Could you check a few things on this model? Use its own coordinates, in mm. A direction names the side the tool comes from. Give positions to 0.01 mm unless a question says otherwise; leave off trailing zeros. Loops run counter-clockwise (first coordinate to the right, second up) from the corner with the lowest first, then second, coordinate; pieces in that order, holes last.
1. Imagine slicing it at D-D (z = -13). List the corners of the cut face in (x, y) for me, plus the area to 3 significant figures.
2. I need wall thicknesses on line 1 along X through (y, z) = (1.75, -7.25) (3 decimals); line 2 along X through (y, z) = (1.15, 7.65) (3 decimals); line 3 along Z through (x, y) = (-15.6, 1.4) (3 decimals). Which ranges of each line are inside material? Lowest first, please.
3. Imagine slicing it at A-A (x = -9). List the corners of the cut face in (y, z) for me, plus the area to 3 significant figures.
4. For P1, Ø1.2, axis at x = -15.6, z = -7.25, coming from the -Y side; P2, Ø1.5, axis at x = 18.5, y = 9, coming from the -Z side; P3, Ø3, axis at x = -14, y = 10, coming from the -Z side, each with a flat end and sliding along its axis, tell me the tip position at first contact or that it passes through.
5. Thinking about a two-plate mould opening in X: for faces 3 (the cylindrical face through (-19.65, 1.23, 15.24)), 4 (the cylindrical face through (19.65, 1.23, -15.24)), 5 (the cylindrical face through (15.05, 1.52, 8.04)), which applies, +X half, -X half, draft (parallel to the pull), parting line (faces both ways), or undercut?
6. Imagine slicing it at C-C (z = 0). List the corners of the cut face in (x, y) for me.
7. Imagine slicing it at B-B (y = 8.25). List the corners of the cut face in (x, z) for me, plus the area to 3 significant figures.
8. For faces 1 (the cylindrical face through (0.18, 9.65, -15.24)), 2 (the cylindrical face through (-14.65, 1.52, -6.86)), which set-ups out of +Z, -Z, +X, -X, +Y, -Y let a thin tool reach every point of the face, with its end or its side?
```python
from build123d import *

# Parameters (mm, degrees)
SKETCH1_W                          = 45
SKETCH1_H                          = 36.5
BOSS_EXTRUDE1_DEPTH                = 12.5
SKETCH2_R                          = 1.375
BOSS_EXTRUDE2_DEPTH                = 1
TAP_DRILL_FOR_M2_5X0_45_TAP1_D     = 2.05
TAP_DRILL_FOR_M2_5X0_45_TAP1_DEPTH = 3
TAP_DRILL_FOR_M2_5X0_45_TAP1_TIP   = 0.615882135
FILLET1_R                          = 10


with BuildPart() as part:
    # Sketch1 → Boss-Extrude1 (new body)
    with BuildSketch(Plane(origin=(0, 0, 0), x_dir=(1, 0, 0), z_dir=(0, 1, 0))):
        Rectangle(SKETCH1_W, SKETCH1_H)
    extrude(amount=BOSS_EXTRUDE1_DEPTH)

    # Sketch2 → Boss-Extrude2 (add)
    with BuildSketch(Plane(origin=(22.5, 0, 0), x_dir=(0, 0, -1), z_dir=(1, 0, 0))):
        with Locations(Location((0, 5.884601179, 0), (0, 0, 180))):
            Circle(SKETCH2_R)
    extrude(amount=BOSS_EXTRUDE2_DEPTH)

    # Tap Drill for M2.5x0.45 Tap1
    with Locations(Plane(origin=(0, 0, 0), x_dir=(-1, 0, 0), z_dir=(0, -1, 0))):
        with Locations((15.6, 7.25), (-14.1, -7.65)):
            Hole(TAP_DRILL_FOR_M2_5X0_45_TAP1_D / 2, depth=TAP_DRILL_FOR_M2_5X0_45_TAP1_DEPTH)
            with Locations((0, 0, -(TAP_DRILL_FOR_M2_5X0_45_TAP1_DEPTH + TAP_DRILL_FOR_M2_5X0_45_TAP1_TIP / 2))):  # 118° drill point
                Cone(0, TAP_DRILL_FOR_M2_5X0_45_TAP1_D / 2, TAP_DRILL_FOR_M2_5X0_45_TAP1_TIP, mode=Mode.SUBTRACT)

    # Fillet1
    # the kernel refuses this fillet: 10 mm, written as the material it takes off along each edge
    with BuildSketch(Plane(origin=(12.5, 2.5, 8.25), x_dir=(1, 0, 0), z_dir=(0, 0, 1))) as fillet1_piece_1_section:
        Polygon((0, 0), (FILLET1_R, 0), (FILLET1_R, FILLET1_R), (0, FILLET1_R), align=None)
    fillet1_piece_1 = extrude(amount=FILLET1_R, mode=Mode.PRIVATE)
    fillet1_piece_1 = fillet1_piece_1 - Plane(origin=(12.5, 2.5, 8.25), x_dir=(-0.7071067811865475, -0.7071067811865475, 0), z_dir=(0, 0, 1)) * Sphere(FILLET1_R, mode=Mode.PRIVATE)
    add(fillet1_piece_1, mode=Mode.SUBTRACT)
    with BuildSketch(Plane(origin=(12.5, 2.5, -8.25), x_dir=(0, 1, 0), z_dir=(1, 0, 0))) as fillet1_piece_2_section:
        Polygon((0, 0), (FILLET1_R, 0), (FILLET1_R, -FILLET1_R), (0, -FILLET1_R), align=None)
    fillet1_piece_2 = extrude(amount=FILLET1_R, mode=Mode.PRIVATE)
    fillet1_piece_2 = fillet1_piece_2 - Plane(origin=(12.5, 2.5, -8.25), x_dir=(0, -0.7071067811865475, 0.7071067811865475), z_dir=(1, 0, 0)) * Sphere(FILLET1_R, mode=Mode.PRIVATE)
    add(fillet1_piece_2, mode=Mode.SUBTRACT)
    with BuildSketch(Plane(origin=(-12.5, 2.5, 8.25), x_dir=(-1, 0, 0), z_dir=(0, 0, 1))) as fillet1_piece_3_section:
        Polygon((0, 0), (FILLET1_R, 0), (FILLET1_R, -FILLET1_R), (0, -FILLET1_R), align=None)
    fillet1_piece_3 = extrude(amount=FILLET1_R, mode=Mode.PRIVATE)
    fillet1_piece_3 = fillet1_piece_3 - Plane(origin=(-12.5, 2.5, 8.25), x_dir=(0.7071067811865475, -0.7071067811865475, 0), z_dir=(0, 0, 1)) * Sphere(FILLET1_R, mode=Mode.PRIVATE)
    add(fillet1_piece_3, mode=Mode.SUBTRACT)
    with BuildSketch(Plane(origin=(-12.5, 2.5, -8.25), x_dir=(0, 1, 0), z_dir=(-1, 0, 0))) as fillet1_piece_4_section:
        Polygon((0, 0), (FILLET1_R, 0), (FILLET1_R, FILLET1_R), (0, FILLET1_R), align=None)
    fillet1_piece_4 = extrude(amount=FILLET1_R, mode=Mode.PRIVATE)
    fillet1_piece_4 = fillet1_piece_4 - Plane(origin=(-12.5, 2.5, -8.25), x_dir=(0, -0.7071067811865475, 0.7071067811865475), z_dir=(-1, 0, 0)) * Sphere(FILLET1_R, mode=Mode.PRIVATE)
    add(fillet1_piece_4, mode=Mode.SUBTRACT)
    with BuildSketch(Plane(origin=(22.5, 12.5, 8.25), x_dir=(0, -1, 0), z_dir=(0, 0, -1))) as fillet1_piece_5_section:
        with BuildLine():
            CenterArc((FILLET1_R, FILLET1_R), FILLET1_R, 180, 90)
            Line((0, FILLET1_R), (0, 0))
            Line((0, 0), (FILLET1_R, 0))
        make_face()
    fillet1_piece_5 = extrude(amount=16.5, mode=Mode.PRIVATE)
    fillet1_piece_5 = fillet1_piece_5 - Plane(origin=(20.212473713, 5.884601179, 0), x_dir=(0, 0, 1), z_dir=(-1, 0, 0)) * Cylinder(1.375, 73, mode=Mode.PRIVATE)
    add(fillet1_piece_5, mode=Mode.SUBTRACT)
    with BuildSketch(Plane(origin=(-12.5, 12.5, 18.25), x_dir=(0, -1, 0), z_dir=(1, 0, 0))) as fillet1_piece_6:
        with BuildLine():
            CenterArc((FILLET1_R, FILLET1_R), FILLET1_R, 180, 90)
            Line((0, FILLET1_R), (0, 0))
            Line((0, 0), (FILLET1_R, 0))
        make_face()
    extrude(amount=25, mode=Mode.SUBTRACT)
    with BuildSketch(Plane(origin=(-22.5, 12.5, -8.25), x_dir=(0, -1, 0), z_dir=(0, 0, 1))) as fillet1_piece_7:
        with BuildLine():
            CenterArc((FILLET1_R, FILLET1_R), FILLET1_R, 180, 90)
            Line((0, FILLET1_R), (0, 0))
            Line((0, 0), (FILLET1_R, 0))
        make_face()
    extrude(amount=16.5, mode=Mode.SUBTRACT)
    with BuildSketch(Plane(origin=(12.5, 12.5, -18.25), x_dir=(0, 0, 1), z_dir=(-1, 0, 0))) as fillet1_piece_8:
        with BuildLine():
            CenterArc((FILLET1_R, -FILLET1_R), FILLET1_R, 90, 90)
            Line((0, -FILLET1_R), (0, 0))
            Line((0, 0), (FILLET1_R, 0))
        make_face()
    extrude(amount=25, mode=Mode.SUBTRACT)
    with BuildSketch(Plane(origin=(-22.5, -25, 18.25), x_dir=(1, 0, 0), z_dir=(0, 1, 0)), Plane(origin=(-22.5, -25, -18.25), x_dir=(0, 0, 1), z_dir=(0, 1, 0))) as fillet1_piece_9:
        with BuildLine():
            CenterArc((FILLET1_R, FILLET1_R), FILLET1_R, 180, 90)
            Line((0, FILLET1_R), (0, 0))
            Line((0, 0), (FILLET1_R, 0))
        make_face()
    extrude(amount=27.5, mode=Mode.SUBTRACT)
    with BuildSketch(Plane(origin=(22.5, -25, 18.25), x_dir=(-1, 0, 0), z_dir=(0, 1, 0)), Plane(origin=(22.5, -25, -18.25), x_dir=(0, 0, 1), z_dir=(0, 1, 0))) as fillet1_piece_10:
        with BuildLine():
            CenterArc((FILLET1_R, -FILLET1_R), FILLET1_R, 90, 90)
            Line((0, -FILLET1_R), (0, 0))
            Line((0, 0), (FILLET1_R, 0))
        make_face()
    extrude(amount=27.5, mode=Mode.SUBTRACT)


solid = part.part
```
Derived:
1. outline: (-21.3, 0) - (21.3, 0) - (21.3, 2.5) arc R8.8 ccw to (12.5, 11.3) - (-12.5, 11.3) arc R8.8 ccw to (-21.3, 2.5) - close
1. area: 448 mm2
2. line 1: x = -22.5 to -16.625, -14.575 to 22.5
2. line 2: x = -22.5 to 13.075, 15.125 to 22.5
2. line 3: z = -17.757 to -8.275, -6.225 to 17.757
3. outline: (0, -18.25) - (2.5, -18.25) arc R10 ccw to (12.5, -8.25) - (12.5, 8.25) arc R10 ccw to (2.5, 18.25) - (0, 18.25) - close
3. area: 413 mm2
4. P1: stops at y = 3.26
4. P2: stops at z = -14.12
4. P3: stops at z = -16.14
5. face 3: -X half
5. face 4: +X half
5. face 5: undercut
6. outline: (-22.5, 0) - (22.5, 0) - (22.5, 2.5) arc R10 ccw to (22.3, 4.51) - (23.5, 4.51) - (23.5, 7.26) - (21.29, 7.26) arc R10 ccw to (12.5, 12.5) - (-12.5, 12.5) arc R10 ccw to (-22.5, 2.5) - close
7. outline: (-20.68, -8.25) arc R8.18 ccw to (-12.5, -16.43) - (12.5, -16.43) arc R8.18 ccw to (20.68, -8.25) - (20.68, 8.25) arc R8.18 ccw to (12.5, 16.43) - (-12.5, 16.43) arc R8.18 ccw to (-20.68, 8.25) - close
7. area: 1,300 mm2
8. face 1: -Z, +X, -X, +Y
8. face 2: -Y
